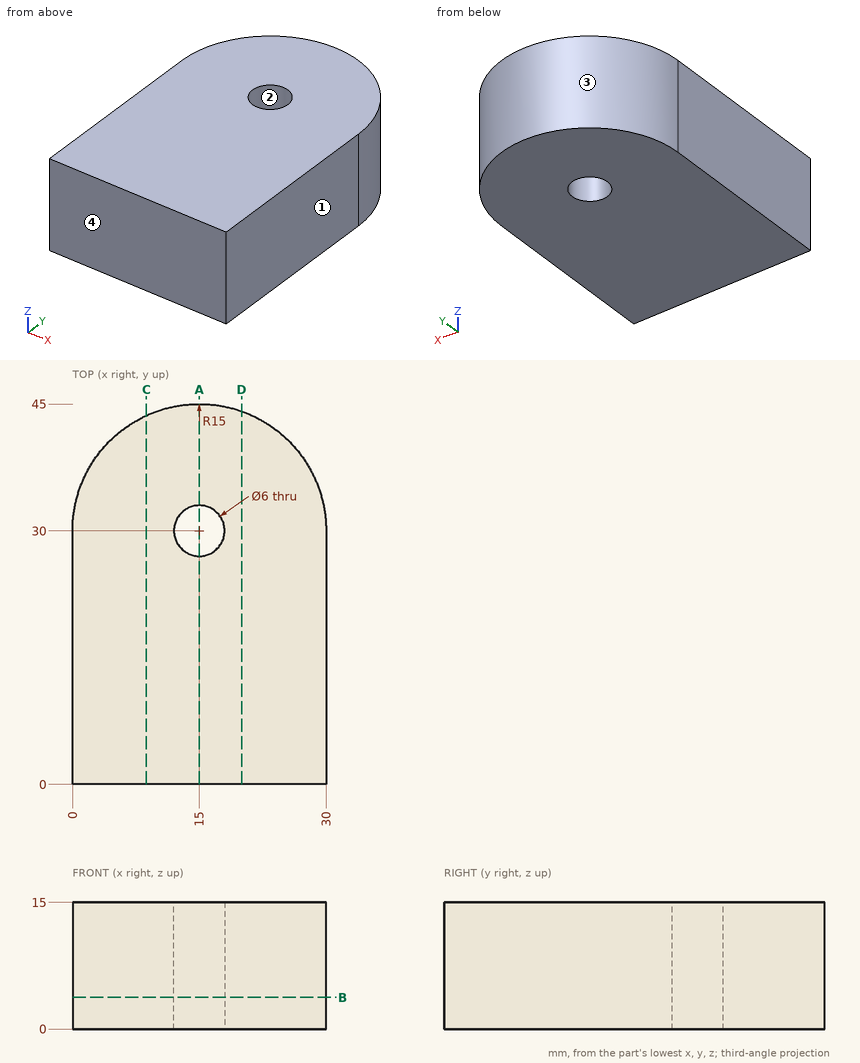
Job drawing, mm, ordinate dimensions from the low corner. One solid piece. Round coordinates to 2 decimals unless told otherwise and drop trailing zeros. Write each loop counter-clockwise with the first axis right and the second up, starting at its lowest first coordinate (ties: lowest second). Pieces come first, ordered by that corner, then holes.
1) Mould opens along Y. For the marked faces 1, 2, 3 and 4 say: +Y half, -Y half, draft (parallel to the pull), parting line (faces both ways), or undercut.
2) Band-saw the part on A-A, the plane x = 15. List the corners of the cut face in (y, z), and give its area (3 significant figures).
3) Drill centre lines: probe 1 along Y at (x, z) = (15, 5); probe 2 along Y at (x, z) = (14.25, 4.75); probe 3 along Y at (x, z) = (20.75, 3.5). Where is each one in solid material? Low to high.
4) Band-saw the part on C-C, the plane x = 8.75. List the corners of the cut face in (y, z), and give its area (3 significant figures).
5) Pin check, flat tips, straight feed: pin 1 (6 mm diameter, centred on y = 20, z = 13, fed in from -X); pin 2 (8 mm diameter, centred on y = 36, z = 1.5, fed in from -X); pin 3 (5 mm diameter, centred on x = 8.5, z = 7, fed in from +Y). Stop position of each tip, or through.
6) Band-saw the part on B-B, the plane z = 3.75. List the corners of the cut face in (x, y).
7) Band-saw the part on D-D, the plane x = 20. List the corners of the cut face in (y, z).
Ans:
1. face 1: draft
1. face 2: undercut
1. face 3: +Y half
1. face 4: -Y half
2. outline: (0, 0) - (27, 0) - (27, 15) - (0, 15) - close; (33, 0) - (45, 0) - (45, 15) - (33, 15) - close
2. area: 585 mm2
3. probe 1: y = 0 to 27, 33 to 45
3. probe 2: y = 0 to 27.1, 32.9 to 44.98
3. probe 3: y = 0 to 43.85
4. outline: (0, 0) - (43.64, 0) - (43.64, 15) - (0, 15) - close
4. area: 655 mm2
5. pin 1: stops at x = 0
5. pin 2: stops at x = 0.13
5. pin 3: stops at y = 44.46
6. outline: (0, 0) - (30, 0) - (30, 30) arc R15 ccw to (0, 30) - close; hole circle Ø6 at (15, 30)
7. outline: (0, 0) - (44.14, 0) - (44.14, 15) - (0, 15) - close
